```python
from build123d import *

# Parameters (mm, degrees)
F0_W        = 80
F0_H        = 279.619
F1_DEPTH    = 40
F2_SIZE2    = 90
F2_SIZE     = 15
F2_2_SIZE2  = 90
F2_2_SIZE   = 15
F3_SIZE     = 8
F4_T        = 2
F5_T1_DEPTH = 86.8350314591


# Not quite as in the source:
# - a fillet or chamfer that OpenCascade refuses, or shapes differently, is made with other operations: its cross-section is extruded or revolved along the edge and cut away or added


with BuildPart() as f1:
    # F0 (on Top) → F1 (new body)
    with BuildSketch(Plane.XY):
        Rectangle(F0_W, F0_H)
    extrude(amount=F1_DEPTH)

    # F2
    f2_edges = [f1.edges().sort_by_distance(p)[0] for p in [
        (0, 139.8095, 40),
    ]]
    f2_side = f1.faces().sort_by_distance((0, 139.8095, 20))[0]
    chamfer(f2_edges, length=F2_SIZE, length2=F2_SIZE2, reference=f2_side)

    # F2#2
    f2_2_edges = [f1.edges().sort_by_distance(p)[0] for p in [
        (0, -139.8095, 40),
    ]]
    f2_2_side = f1.faces().sort_by_distance((0, -139.8095, 20))[0]
    chamfer(f2_2_edges, length=F2_2_SIZE, length2=F2_2_SIZE2, reference=f2_2_side)

    # F3
    f3_edges = [f1.edges().sort_by_distance(p)[0] for p in [
        (-40, -94.8095, 32.5),
        (40, -94.8095, 32.5),
        (40, 94.8095, 32.5),
        (-40, 94.8095, 32.5),
    ]]
    chamfer(f3_edges, length=F3_SIZE)

    # F4
    f4_openings = [f1.faces().sort_by_distance(p)[0] for p in [
        (0, 0, 0),
    ]]
    offset(amount=F4_T, openings=f4_openings, kind=Kind.INTERSECTION)

    # F5: fillet of radius 5 on 2 edges, made by hand

    # F5_s2 → F5_t1 (cut)
    with BuildSketch(Plane.YZ.offset(-43.4175157295)):
        with BuildLine():
            ThreePointArc((-141.8095, 22.4586187349), (-140.6245999124, 25.6904932155), (-137.6314949365, 27.390588354))
            Line((-137.6314949365, 27.390588354), (-141.8095, 26.6942541768))
            Line((-141.8095, 26.6942541768), (-141.8095, 22.4586187349))
        make_face()
        with BuildLine():
            ThreePointArc((141.8095, 22.4586187349), (140.6245999124, 25.6904932155), (137.6314949365, 27.390588354))
            Line((137.6314949365, 27.390588354), (141.8095, 26.6942541768))
            Line((141.8095, 26.6942541768), (141.8095, 22.4586187349))
        make_face()
    extrude(amount=F5_T1_DEPTH, mode=Mode.SUBTRACT)


solid = f1.part
```
The listing builds one solid part. Answer for the finished solid, in the listing's coordinates (mm). A direction names the side the tool comes from. Round coordinates to 2 decimals unless told otherwise and drop trailing zeros. Order: outer loops, then holes, each group sorted by start corner. A loop starts at its lowest first (then second) coordinate and runs counter-clockwise, first axis right, second up. Notation, with made-up numbers: (74, 30.5) - (111, 30.5) arc R32 cw to (111, 60.5) - close; hole circle Ø11 at (52.25, -13.75). An arc over 180 degrees is marked (long way). Put each result on its own line as item: value. Start each with the question number.
(1) Find section C-C (y = 71). Give the vertices of the cut face in (x, z), plus the area to 3 significant figures.
(2) Find section A-A (x = 26.5). Give the vertices of the cut face in (y, z), plus the area to 3 significant figures.
(3) For faces 1 (the flat face through (-1, 139.81, 12)), 2 (the flat face through (-0.46, -93.19, 34.798)), determine the directions among +Z, -Z, +X, -X, +Y, -Y from which every point of the face is accessible in a straight line to the end or side of a thin tool.
(4) Determine the mould class of faces 3 (the flat face through (-0.46, 93.19, 34.798)), 4 (the flat face through (-35.94, -87.52, 29.72)), 5 (the flat face through (-41, 1, 0)) for opening direction Y: released by +Y, released by -Y, zero draft, split by the parting line, or undercut.
(5) Given P1, Ø3, axis at x = -3, y = -109, coming from the +Z side, flat-ended and moving along its own axis, determine where the tip first touches the part or whether it passes through.
(6) Find section D-D (z = 32.5). Give the vertices of the cut face in (x, y), plus the area to 3 significant figures.
(7) Straight lines are drawn through the part: probe 1 along Y at (x, z) = (-29.5, 22); probe 2 along X at (y, z) = (73, 6); probe 3 along Z at (x, y) = (11.5, -1.5). For each, find the intervals that lie inside material, in ascending order. Write a range as from..to.
(8) Find section B-B (z = 12). Give the vertices of the cut face in (x, y).
Reply:
1. outline: (-42, 0) - (-40, 0) - (-40, 28.36) - (-32, 36.47) - (32, 36.47) - (40, 28.36) - (40, 0) - (42, 0) - (42, 29.2) - (32.83, 38.5) - (-32.83, 38.5) - (-42, 29.2) - close
1. area: 296 mm^2
2. outline: (-141.81, 0) - (-139.81, 0) - (-139.81, 25) - (-49.81, 40) - (49.81, 40) - (139.81, 25) - (139.81, 0) - (141.81, 0) - (141.81, 22.46) arc R5 ccw to (137.63, 27.39) - (49.98, 42) - (-49.98, 42) - (-137.63, 27.39) arc R5 ccw to (-141.81, 22.46) - close
2. area: 664 mm^2
3. face 1: -Z
3. face 2: +Z, +X, -X, -Y
4. face 3: released by +Y
4. face 4: undercut
4. face 5: zero draft
5. P1: z = 32.41
6. outline: (-42, -51.19) - (-32.83, -106.98) - (32.83, -106.98) - (42, -51.19) - (42, 51.19) - (32.83, 106.98) - (-32.83, 106.98) - (-42, 51.19) - close; hole (-40, -46.15) - (-32, -94.81) - (32, -94.81) - (40, -46.15) - (40, 46.15) - (32, 94.81) - (-32, 94.81) - (-40, 46.15) - close
6. area: 2,560 mm^2
7. probe 1: -141.81..-139.81, 139.81..141.81
7. probe 2: -42..-40, 40..42
7. probe 3: 40..42
8. outline: (-42, -141.81) - (42, -141.81) - (42, 141.81) - (-42, 141.81) - close; hole (-40, -139.81) - (40, -139.81) - (40, 139.81) - (-40, 139.81) - close
